```python
from build123d import *

# Parameters (mm, degrees)
SKETCH1_R          = 23.8125
WHEEL_BODY_DEPTH   = 5.715
SKETCH2_R          = 2.8
C24T_SPLINE_DEPTH  = 3.4544
SKETCH3_R          = 1.905
CUT_EXTRUDE2_DEPTH = 35.157452152


with BuildPart() as part:
    # Sketch1 → Wheel Body (new body)
    with BuildSketch(Plane(origin=(0, 0, 0), x_dir=(0, 0, -1), z_dir=(1, 0, 0))):
        Circle(SKETCH1_R)
    extrude(amount=WHEEL_BODY_DEPTH)

    # Sketch2 → C24T Spline (cut)
    with BuildSketch(Plane(origin=(0, 0, 0), x_dir=(0, 0, -1), z_dir=(1, 0, 0))):
        Circle(SKETCH2_R)
    extrude(amount=C24T_SPLINE_DEPTH, mode=Mode.SUBTRACT)

    # Sketch3 → Cut-Extrude2 (cut, through all)
    with BuildSketch(Plane.ZY):
        with Locations((-10.429406727, 11.349688472)):
            Circle(SKETCH3_R)
        with Locations((7.571331259, 13.426201847)):
            Circle(SKETCH3_R)
        with Locations((15.108746785, -3.05183939)):
            Circle(SKETCH3_R)
        with Locations((1.766387782, -15.312342319)):
            Circle(SKETCH3_R)
        with Locations((-14.017059099, -6.41170861)):
            Circle(SKETCH3_R)
    extrude(amount=-CUT_EXTRUDE2_DEPTH, mode=Mode.SUBTRACT)


solid = part.part
```
Input: part model. Units: mm. Frame: model coordinates. A direction names the side the tool comes from. Round coordinates to 2 decimals unless told otherwise and drop trailing zeros. Order: outer loops, then holes, each group sorted by start corner. A loop starts at its lowest first (then second) coordinate and runs counter-clockwise, first axis right, second up. Notation, with made-up numbers: (43, 80) - (73, 80) arc R21 cw to (73, 98) - close; hole circle Ø4 at (64.25, 41.25). An arc over 180 degrees is marked (long way). Answer in a Markdown table with one row per item.
Item 1: Pin query (flat end, axial travel): pin 1 (3 mm diameter, centred on y = 1.5, z = 0, fed in from -X); pin 2 (3.5 mm diameter, centred on y = -3.05, z = 15.11, fed in from +X); pin 3 (3 mm diameter, centred on x = 1.5, y = -14.5, fed in from +Z). Return the tip coordinate at first contact, or that it passes through.
Model answer:
| item | result |
|---|---|
| pin 1 | stops at x = 0 |
| pin 2 | passes through |
| pin 3 | stops at z = 19.95 |
Item 2: Section query D-D (x = 0.65). Return the cut outline in (y, z) (1 decimal).
Model answer:
| item | result |
|---|---|
| outline | circle Ø47.6 at (0, 0); hole circle Ø3.8 at (-15.3, 1.8); hole circle Ø3.8 at (-6.4, -14); hole circle Ø3.8 at (-3.1, 15.1); hole circle Ø5.6 at (0, 0); hole circle Ø3.8 at (11.3, -10.4); hole circle Ø3.8 at (13.4, 7.6) |
Item 3: Section query A-A (y = 0). Return the cut outline in (x, z) (1 decimal).
Model answer:
| item | result |
|---|---|
| outline | (0, -23.8) - (5.7, -23.8) - (5.7, 23.8) - (0, 23.8) - (0, 2.8) - (3.5, 2.8) - (3.5, -2.8) - (0, -2.8) - close |
Item 4: Line query: line 1 (Y direction, x = 1.3, z = -10.5); line 2 (Y direction, x = 1.2, z = -2); line 3 (Z direction, x = 3.25, y = -2.5). Output: solid intervals per line, ascending.
Model answer:
| item | result |
|---|---|
| line 1 | y = -21.37 to 9.45, 13.25 to 21.37 |
| line 2 | y = -23.73 to -1.96, 1.96 to 23.73 |
| line 3 | z = -23.68 to -1.26, 1.26 to 13.29, 16.93 to 23.68 |
Item 5: Section query B-B (z = 8). Return the cut outline in (x, y) (3 decimals), then the cut area to 3 significant figures.
Model answer:
| item | result |
|---|---|
| outline | (0, -22.428) - (5.715, -22.428) - (5.715, 11.57) - (0, 11.57) - close; (0, 15.282) - (5.715, 15.282) - (5.715, 22.428) - (0, 22.428) - close |
| area | 235 mm² |
Item 6: Reachability of faces 5 (the cylindrical face through (1.7, 0.1, 2.8)), 6 (the cylindrical face through (2.82, 13.51, 5.67)) from +Z, -Z, +X, -X, +Y, -Y: full face, straight path, thin tool, end or side. Return the list, or none.
Model answer:
| item | result |
|---|---|
| face 5 | -X |
| face 6 | +X, -X |
Item 7: Mould query, pull axis Y, two halves, no side actions, for faces 1 (the flat face through (5.715, 0, 0)), 2 (the cylindrical face through (2.82, 11.92, -8.61)), 3 (the cylindrical face through (2.817, -14.49, 18.897)), 4 (the flat face through (3.454, 0, 0)). Classes: released by +Y, released by -Y, zero draft, split by the parting line, or undercut.
Model answer:
| item | result |
|---|---|
| face 1 | zero draft |
| face 2 | undercut |
| face 3 | split by the parting line |
| face 4 | undercut |
Item 8: Section query C-C (y = -14.5). Return the cut outline in (x, z) (1 decimal).
Model answer:
| item | result |
|---|---|
| outline | (0, -18.9) - (5.7, -18.9) - (5.7, 0) - (0, 0) - close; (0, 3.5) - (5.7, 3.5) - (5.7, 18.9) - (0, 18.9) - close |
